Work out the finished part from the listing and answer in its coordinate system (mm). A direction names the side the tool comes from. Round coordinates to 2 decimals unless told otherwise and drop trailing zeros. Loops run counter-clockwise (first coordinate to the right, second up) from the corner with the lowest first, then second, coordinate; pieces in that order, holes last.
```python
from build123d import *

# Parameters (mm, degrees)
SKETCH_1_W          = 40
SKETCH_1_H          = 15
SKETCH_1_R          = 1.5
EXTRUDE_1_DEPTH     = 3
SKETCH_5_R          = 1.5
CUT_EXTRUDE_3_DEPTH = 8
SKETCH_8_R          = 2.999642866
CUT_EXTRUDE_4_DEPTH = 15
SKETCH_9_R          = 1.5
CUT_EXTRUDE_5_DEPTH = 15


with BuildPart() as part:
    # 草图1 → 凸台-拉伸1 (new body)
    with BuildSketch(Plane.XY):
        Rectangle(SKETCH_1_W, SKETCH_1_H)
        with Locations((4.95, 4.95)):
            Circle(SKETCH_1_R, mode=Mode.SUBTRACT)
        with Locations((4.95, -4.95)):
            Circle(SKETCH_1_R, mode=Mode.SUBTRACT)
        with Locations((-4.95, -4.95)):
            Circle(SKETCH_1_R, mode=Mode.SUBTRACT)
        with Locations((-4.95, 4.95)):
            Circle(SKETCH_1_R, mode=Mode.SUBTRACT)
    extrude(amount=EXTRUDE_1_DEPTH)

    # 草图3 → 放样1 section 0
    with BuildSketch(Plane.XY.offset(43)):
        with BuildLine():
            Line((-5.5, -5.5), (5.5, -5.5))
            Line((5.5, -5.5), (5.5, 5.5))
            Line((5.5, 5.5), (-5.5, 5.5))
            Line((-5.5, 5.5), (-5.5, -5.5))
        make_face()
    # 草图2 → 放样1 section 1
    with BuildSketch(Plane.XY.offset(3)):
        with BuildLine():
            Line((-7.5, -7.5), (7.5, -7.5))
            Line((7.5, -7.5), (7.5, 7.5))
            Line((7.5, 7.5), (-7.5, 7.5))
            Line((-7.5, 7.5), (-7.5, -7.5))
        make_face()
    loft()

    # 草图5 → 切除-拉伸3 (cut)
    with BuildSketch(Plane(origin=(0, 0, 0), x_dir=(-1, 0, 0), z_dir=(0, 0, -1))):
        with Locations((4.95, -4.95)):
            Circle(SKETCH_5_R)
        with Locations((4.95, 4.95)):
            Circle(SKETCH_5_R)
        with Locations((-4.95, 4.95)):
            Circle(SKETCH_5_R)
        with Locations((-4.95, -4.95)):
            Circle(SKETCH_5_R)
    extrude(amount=-CUT_EXTRUDE_3_DEPTH, mode=Mode.SUBTRACT)

    # 草图8 → 切除-拉伸4 (cut)
    with BuildSketch(Plane.XY.offset(43)):
        Circle(SKETCH_8_R)
    extrude(amount=-CUT_EXTRUDE_4_DEPTH, mode=Mode.SUBTRACT)

    # 草图9 → 切除-拉伸5 (cut)
    with BuildSketch(Plane(origin=(0, 0, 0), x_dir=(-1, 0, 0), z_dir=(0, 0, -1))):
        with Locations((-14.848989873, -4.95)):
            Circle(SKETCH_9_R)
        with Locations((-14.848989873, 4.949494937)):
            Circle(SKETCH_9_R)
        with Locations((14.849494937, 4.949494937)):
            Circle(SKETCH_9_R)
        with Locations((14.849494937, -4.95)):
            Circle(SKETCH_9_R)
    extrude(amount=-CUT_EXTRUDE_5_DEPTH, mode=Mode.SUBTRACT)


solid = part.part
```
1. Consider probe 1 along X at (y, z) = (4.95, 4.4); probe 2 along X at (y, z) = (-4.95, 6.25); probe 3 along Y at (x, z) = (-4.95, 4.75). Determine where each line is inside the solid, lowest interval first.
Answer key:
probe 1: x = -7.43 to -6.45, -3.45 to 3.45, 6.45 to 7.43
probe 2: x = -7.34 to -6.45, -3.45 to 3.45, 6.45 to 7.34
probe 3: y = -7.41 to -6.45, -3.45 to 3.45, 6.45 to 7.41
2. Find section A-A (x = 17). Write down the section's boundary in (y, z), then the cut area to 3 significant figures.
Answer key:
outline: (-7.5, 0) - (7.5, 0) - (7.5, 3) - (-7.5, 3) - close
area: 45.0 mm2
3. Which of the six approach directions +Z, -Z, +X, -X, +Y, -Y give full straight-line access (tool end or side, diameter ignored) to faces 1 (the face through (-14, 0, 3)), 2 (the face through (0, 0, 0)), 3 (the face through (2.86, 0.9, 35.61)), 4 (the face through (5, 5, 8)), 5 (the face through (14, 0, 3))?
Answer key:
face 1: +Z, -X, +Y, -Y
face 2: -Z, +X, -X, +Y, -Y
face 3: +Z
face 4: -Z
face 5: +Z, +X, +Y, -Y
4. Find section B-B (z = 5.5). Give the number of separate pieces and of enclosed holes in the cut face, then the cut area to 3 significant figures.
Answer key:
separate pieces: 1
enclosed holes: 4
area: 189 mm2
5. Determine the mould class of faces 6 (the face through (5, -5, 8)), 7 (the face through (20, 0, 1)), 8 (the face through (-5, 5, 8)), 9 (the face through (-20, 0, 1)) for opening direction X: +X half, -X half, draft (parallel to the pull), parting line (faces both ways), or undercut.
Answer key:
face 6: undercut
face 7: +X half
face 8: undercut
face 9: -X half
6. Given pin 1 (12 mm diameter, centred on x = 11, z = 24.5, fed in from +Y); pin 2 (3 mm diameter, centred on y = -4.5, z = 33, fed in from +X) (3 decimals); pin 3 (0.9 mm diameter, centred on x = -5.5, y = 4.5, fed in from -Z), each flat-ended and moving along its own axis, determine where each tip first touches the part or whether it passes through.
Answer key:
pin 1: stops at y = 6.63
pin 2: stops at x = 6.075
pin 3: stops at z = 8
